Check sheet for the modelled part. Datum: model origin and axes. Units: mm. Face numbers are marked on the shaded views. A direction names the side the tool comes from. Give positions to 0.01 mm unless a question says otherwise; leave off trailing zeros. Order: outer loops, then holes, each group sorted by start corner. A loop starts at its lowest first (then second) coordinate and runs counter-clockwise, first axis right, second up. Notation, with made-up numbers: (31, -21.5) -> (39, -21.5) arc R28 cw to (39, -3.5) -> close; hole circle Ø5 at (27, 67.5). An arc over 180 degrees is marked (long way). Answer in a Markdown table with one row per item. Add a question column.
(1) Release check for a two-part mould opening along X. For the marked faces 3, 4 and 5 record: released by +X, released by -X, zero draft, split by the parting line, or undercut.
(2) Cross-section at B-B (z = 0). Record the cut outline in (x, y) (3 decimals), then the cut area to 3 significant figures.
(3) Set-up check for the marked faces 1 and 2: record each of +Z, -Z, +X, -X, +Y, -Y from which the full face is reachable in a straight line by a thin tool's end or side.
(4) Cross-section at A-A (x = 0). Record the cut outline in (y, z) (3 decimals).
(5) Go/stop test with flat-tipped pins: pin 1 (4 mm diameter, centred on y = -3.5, z = -12, fed in from +X); pin 2 (7 mm diameter, centred on x = 0, z = 0, fed in from +Y); pin 3 (4 mm diameter, centred on y = -6.5, z = -11.5, fed in from -X); pin 4 (2 mm diameter, centred on y = -5, z = -1, fed in from -X). Record where each tip stops, or that it passes through.
(6) Thickness scan on L1, parallel to Z at x = 0, y = -2 (3 decimals); L2, parallel to Z at x = 0, y = -3 (3 decimals); L3, parallel to Y at x = 4.25, z = -10.75. Record the ranges inside material, lowest first. Write a range as [from, to].
(7) Cross-section at C-C (y = -1). Record the cut outline in (x, z) (3 decimals).
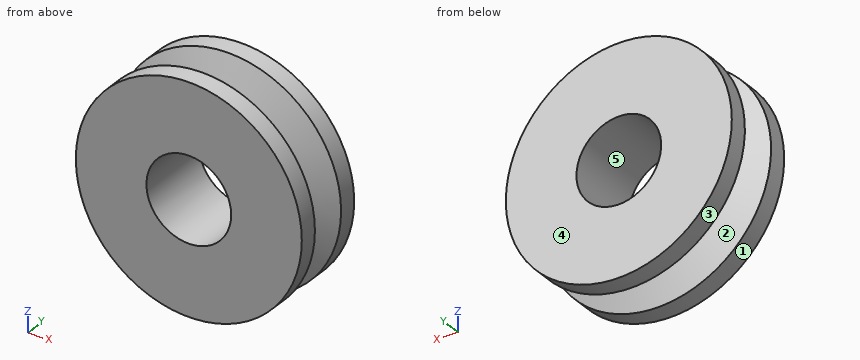
```python
from build123d import *

# Parameters (mm, degrees)
F0_R     = 15
F0_R_2   = 5.625
F1_DEPTH = 10


with BuildPart() as f1:
    # F0 (on Front) → F1 (new body)
    with BuildSketch(Plane.XZ):
        Circle(F0_R)
        Circle(F0_R_2, mode=Mode.SUBTRACT)
    extrude(amount=F1_DEPTH)

    # F3 (on offset) → F4 (revolve, cut)
    with BuildSketch(Plane.YZ):
        Polygon((-2.5, 15), (-7.5, 15), (-5, 8.964466), align=None)
    revolve(axis=Axis((0, 0, 0), (0, 1, 0)), mode=Mode.SUBTRACT)


solid = f1.part
```
Answer below:
| question | item | result |
|---|---|---|
| 1 | face 3 | split by the parting line |
| 1 | face 4 | zero draft |
| 1 | face 5 | undercut |
| 2 | outline | (-15, -10) -> (-5.625, -10) -> (-5.625, 0) -> (-15, 0) -> (-15, -2.5) -> (-8.964, -5) -> (-15, -7.5) -> close; (5.625, -10) -> (15, -10) -> (15, -7.5) -> (8.964, -5) -> (15, -2.5) -> (15, 0) -> (5.625, 0) -> close |
| 2 | area | 157 mm² |
| 3 | face 1 | +Y, -Y |
| 3 | face 2 | none |
| 4 | outline | (-10, -15) -> (-7.5, -15) -> (-5, -8.964) -> (-2.5, -15) -> (0, -15) -> (0, -5.625) -> (-10, -5.625) -> close; (-10, 5.625) -> (0, 5.625) -> (0, 15) -> (-2.5, 15) -> (-5, 8.964) -> (-7.5, 15) -> (-10, 15) -> close |
| 5 | pin 1 | stops at x = 10.93 |
| 5 | pin 2 | passes through |
| 5 | pin 3 | stops at x = -11.38 |
| 5 | pin 4 | stops at x = -11.34 |
| 6 | L1 | z = [-15, -5.625], [5.625, 15] |
| 6 | L2 | z = [-13.793, -5.625], [5.625, 13.793] |
| 6 | L3 | y = [-10, -6.07], [-3.93, 0] |
| 7 | outline | circle Ø30 at (0, 0); hole circle Ø11.25 at (0, 0) |
